Input: part model. Units: mm. Frame: model coordinates. A direction names the side the tool comes from. Coordinates: 2 decimals unless noted, no trailing zeros. Write each loop counter-clockwise with the first axis right and the second up, starting at its lowest first coordinate (ties: lowest second). Pieces come first, ordered by that corner, then holes. Notation, with made-up numbers: (32, 41) - (37, 41) arc R17 cw to (37, 60) - close; hole circle Ø11 at (49, -38). An arc over 180 degrees is marked (long way). Put each result on its own line as item: value. Start each with the question number.
1. Cut plane B-B, the plane x = 16.5. Return loops of the section in (y, z), and give its area (3 significant figures).
2. Pull-direction query (Z, two-part tool) for faces 4 (the cylindrical face through (-16.99, -38.99, 27.15)), 5 (the cylindrical face through (-19.52, 19.37, 0.99)), 6 (the flat face through (4, 15, 20)); classes: released by +Z, released by -Z, zero draft, split by the parting line, or undercut.
3. Pin query (flat end, axial travel): pin 1 (3.5 mm diameter, centred on x = 19, y = -20, fed in from +Z); pin 2 (8 mm diameter, centred on y = 17.5, z = 5.5, fed in from +X); pin 3 (7 mm diameter, centred on x = -20, y = 15, fed in from +Z). Return the tip coordinate at first contact, or that it passes through.
4. Cut plane C-C, the plane y = 25. Return loops of the section in (x, z).
5. Cut plane A-A, the plane y = 51. Return loops of the section in (x, z).
6. Line query: line 1 (Z direction, x = 8.5, y = -33); line 2 (Y direction, x = 29.5, z = -9.5); line 3 (Y direction, x = -5.5, z = 11). Output: solid intervals per line, ascending.
7. Cut plane D-D, the plane z = 23. Return loops of the section in (x, y).
8. Access query for faces 1 (the cylindrical face through (-14.7, 22.3, 5.9)), 2 (the flat face through (-4, 10, 20)), 3 (the flat face through (10, 0, 12)). Directions: +Z, -Z, +X, -X, +Y, -Y. A direction counts if a zero-diameter tool reaches every point of the face in a straight line with its end or side. Return the directions, or none.
from build123d import *

# Parameters (mm, degrees)
SKETCH1_R                = 5.5
BOSS_EXTRUDE1_DEPTH      = 10
SKETCH1_3_R              = 5.5
SKETCH1_3_R_2            = 2.5
BOSS_EXTRUDE2_DEPTH      = 2
SKETCH1_4_R              = 2.5
BOSS_EXTRUDE3_DEPTH      = 5
BOSS_EXTRUDE4_DEPTH      = 5
SKETCH4_W                = 20
SKETCH4_H                = 80
BOSS_EXTRUDE5_DEPTH      = 20
SKETCH5_W                = 20
SKETCH5_H                = 2
BOSS_EXTRUDE6_DEPTH      = 10
BOSS_EXTRUDE6_DEPTH_BACK = 30
SKETCH7_W                = 5
SKETCH7_H                = 10
CUT_EXTRUDE1_DEPTH       = 78
FILLET1_R                = 10
SKETCH9_W                = 10
SKETCH9_H                = 5
CUT_EXTRUDE2_DEPTH       = 2.5
SKETCH14_R               = 1.5
BOSS_EXTRUDE8_DEPTH      = 3
SKETCH16_W               = 10
SKETCH16_H               = 5
CUT_EXTRUDE4_DEPTH       = 2.5


with BuildPart() as part:
    # Sketch1 → Boss-Extrude1 (new body)
    with BuildSketch(Plane.XY):
        with BuildLine():
            Line((31.5, 0), (31.5, 40))
            Line((31.5, 40), (-31.5, 40))
            Line((-31.5, 40), (-31.5, 0))
            ThreePointArc((-31.5, 0), (0, -31.5), (31.5, 0))
        make_face()
        with Locations((17.67766953, -17.67766953)):
            Circle(SKETCH1_R, mode=Mode.SUBTRACT)
        with Locations((-17.67766953, -17.67766953)):
            Circle(SKETCH1_R, mode=Mode.SUBTRACT)
        with Locations((-17.67766953, 17.67766953)):
            Circle(SKETCH1_R, mode=Mode.SUBTRACT)
        with Locations((17.67766953, 17.67766953)):
            Circle(SKETCH1_R, mode=Mode.SUBTRACT)
    extrude(amount=BOSS_EXTRUDE1_DEPTH)

    # Sketch1<3> → Boss-Extrude2 (add)
    with BuildSketch(Plane.XY):
        with Locations((17.67766953, 17.67766953)):
            Circle(SKETCH1_3_R)
        with Locations((17.67766953, 17.67766953)):
            Circle(SKETCH1_3_R_2, mode=Mode.SUBTRACT)
        with Locations((17.67766953, -17.67766953)):
            Circle(SKETCH1_3_R)
        with Locations((17.67766953, -17.67766953)):
            Circle(SKETCH1_3_R_2, mode=Mode.SUBTRACT)
        with Locations((-17.67766953, -17.67766953)):
            Circle(SKETCH1_3_R)
        with Locations((-17.67766953, -17.67766953)):
            Circle(SKETCH1_3_R_2, mode=Mode.SUBTRACT)
        with Locations((-17.67766953, 17.67766953)):
            Circle(SKETCH1_3_R)
        with Locations((-17.67766953, 17.67766953)):
            Circle(SKETCH1_3_R_2, mode=Mode.SUBTRACT)
    extrude(amount=BOSS_EXTRUDE2_DEPTH)

    # Sketch1<4> → Boss-Extrude3 (add)
    with BuildSketch(Plane.XY):
        with Locations((0, 25)):
            Circle(SKETCH1_4_R)
    extrude(amount=-BOSS_EXTRUDE3_DEPTH)

    # Sketch2 → Boss-Extrude4 (add)
    with BuildSketch(Plane(origin=(0, 40, 0), x_dir=(1, 0, 0), z_dir=(0, 1, 0))):
        Polygon((-32.5, -10), (31.5, -10), (32.5, -10), (32.5, 15), (-32.5, 15), align=None)
    extrude(amount=-BOSS_EXTRUDE4_DEPTH)

    # Sketch4 → Boss-Extrude5 (add)
    with BuildSketch(Plane.XY.offset(10)):
        Rectangle(SKETCH4_W, SKETCH4_H)
    extrude(amount=BOSS_EXTRUDE5_DEPTH)

    # Sketch5 → Boss-Extrude6 (add, two sides)
    with BuildSketch(Plane(origin=(10, 0, 0), x_dir=(0, 0, -1), z_dir=(1, 0, 0))) as boss_extrude6_sk:
        with Locations((-20, -39)):
            Rectangle(SKETCH5_W, SKETCH5_H)
    extrude(amount=BOSS_EXTRUDE6_DEPTH)
    extrude(boss_extrude6_sk.sketch, amount=-BOSS_EXTRUDE6_DEPTH_BACK)

    # Sketch7 → Cut-Extrude1 (cut)
    with BuildSketch(Plane(origin=(0, 40, 0), x_dir=(1, 0, 0), z_dir=(0, 1, 0))):
        with Locations((-7.5, -20)):
            Rectangle(SKETCH7_W, SKETCH7_H)
        with Locations((7.5, -20)):
            Rectangle(SKETCH7_W, SKETCH7_H)
    extrude(amount=-CUT_EXTRUDE1_DEPTH, mode=Mode.SUBTRACT)

    # Fillet1
    fillet1_edges = [part.edges().sort_by_distance(p)[0] for p in [
        (-20, -39, 30),
        (20, -39, 30),
    ]]
    fillet(fillet1_edges, radius=FILLET1_R)

    # Sketch9 → Cut-Extrude2 (cut)
    with BuildSketch(Plane(origin=(5, 0, 0), x_dir=(0, 0, -1), z_dir=(1, 0, 0))):
        with Locations((-20, 12.5)):
            Rectangle(SKETCH9_W, SKETCH9_H)
    extrude(amount=-CUT_EXTRUDE2_DEPTH, mode=Mode.SUBTRACT)

    # Sketch14 → Boss-Extrude8 (add)
    with BuildSketch(Plane(origin=(0, 0, -15), x_dir=(-1, 0, 0), z_dir=(0, 0, -1))):
        with BuildLine():
            Line((32.5, 62), (-32.5, 62))
            ThreePointArc((-32.5, 62), (-43.5, 51), (-32.5, 40))
            Line((-32.5, 40), (32.5, 40))
            ThreePointArc((32.5, 40), (43.5, 51), (32.5, 62))
        make_face()
        with Locations((-22, 51)):
            Circle(SKETCH14_R, mode=Mode.SUBTRACT)
        with Locations((22, 51)):
            Circle(SKETCH14_R, mode=Mode.SUBTRACT)
    extrude(amount=-BOSS_EXTRUDE8_DEPTH)

    # Sketch16 → Cut-Extrude4 (cut)
    with BuildSketch(Plane.ZY.offset(5)):
        with Locations((20, 12.5)):
            Rectangle(SKETCH16_W, SKETCH16_H)
    extrude(amount=-CUT_EXTRUDE4_DEPTH, mode=Mode.SUBTRACT)


solid = part.part
Report:
1. outline: (-40, 10) - (-38, 10) - (-38, 27.6) - (-40, 27.6) - close; (-26.83, 0) - (-19.88, 0) - (-19.88, 2) - (-23.05, 2) - (-23.05, 10) - (-26.83, 10) - close; (-15.47, 0) - (15.47, 0) - (15.47, 2) - (12.31, 2) - (12.31, 10) - (-12.31, 10) - (-12.31, 2) - (-15.47, 2) - close; (19.88, 0) - (35, 0) - (35, -15) - (62, -15) - (62, -12) - (40, -12) - (40, 10) - (23.05, 10) - (23.05, 2) - (19.88, 2) - close
1. area: 655 mm^2
2. face 4: released by +Z
2. face 5: zero draft
2. face 6: undercut
3. pin 1: stops at z = 2
3. pin 2: stops at x = 31.5
3. pin 3: stops at z = 10
4. outline: (-31.5, 0) - (-2.5, 0) - (-2.5, -5) - (2.5, -5) - (2.5, 0) - (31.5, 0) - (31.5, 10) - (10, 10) - (10, 15) - (5, 15) - (5, 25) - (10, 25) - (10, 30) - (-10, 30) - (-10, 25) - (-5, 25) - (-5, 15) - (-10, 15) - (-10, 10) - (-31.5, 10) - close
5. outline: (-43.5, -15) - (-23.5, -15) - (-23.5, -12) - (-43.5, -12) - close; (-20.5, -15) - (20.5, -15) - (20.5, -12) - (-20.5, -12) - close; (23.5, -15) - (43.5, -15) - (43.5, -12) - (23.5, -12) - close
6. line 1: z = 10 to 15, 25 to 30
6. line 2: y = 35 to 40
6. line 3: y = -40 to 40
7. outline: (-19.54, -40) - (19.54, -40) - (19.54, -38) - (5, -38) - (5, 10) - (2.5, 10) - (2.5, 15) - (5, 15) - (5, 40) - (-5, 40) - (-5, 15) - (-2.5, 15) - (-2.5, 10) - (-5, 10) - (-5, -38) - (-19.54, -38) - close
8. face 1: +Z
8. face 2: -X
8. face 3: +Z, +X, +Y
